Part model, mm, in its own coordinate system. A direction names the side the tool comes from. Coordinates: 2 decimals unless noted, no trailing zeros. Loops run counter-clockwise (first coordinate to the right, second up) from the corner with the lowest first, then second, coordinate; pieces in that order, holes last. Notation, with made-up numbers: M 79,29.5 L 111,29.5 A9 ccw 111,33.5 Z; hole C 35,39.5 d5. An arc over 180 degrees is marked long. Use a Markdown table: item, result. Add a question column.
1) Band-saw the part on D-D (y = 7.25). List the corners of the cut face in (x, z).
2) Band-saw the part on A-A (x = 0). List the corners of the cut face in (y, z), plus the area to 3 significant figures.
3) Pin check, flat tips, straight feed: pin 1 Ø1.5 at (y, z) = (7.5, -7) entering from +X; pin 2 Ø3 at (y, z) = (2.5, -3.5) entering from -X; pin 3 Ø4 at (x, z) = (0, -6.5) entering from +Y; pin 4 Ø4 at (x, z) = (0, 8.3) entering from +Y. Stop position of each tip, or through.
4) Pull direction Z, two halves, no side cores. Call faces 1 (the cylindrical face through (4.336, 8.874, 19.524)), 2 (the cylindrical face through (6.586, 15.042, -10.329)), 3 (the flat face through (13.42, 20, -5.25)): released by +Z, released by -Z, zero draft, split by the parting line, or undercut.
5) Band-saw the part on B-B (y = 14.75). List the corners of the cut face in (x, z), plus the area to 3 significant figures.
6) Wall check: probe 1 along Z at (x, y) = (0, 9); probe 2 along Z at (x, y) = (0, 15); probe 3 along X at (y, z) = (17.75, -0.5). Give the ranges that are in metal, low to high. Write a range as from..to.
7) Tool access for faces 4 (the cylindrical face through (-0.867, 15.944, -3.905)), 5 (the flat face through (0, 0, 0)): list every direction of +Z, -Z, +X, -X, +Y, -Y with a clear straight run to the whole face (end or side of a thin tool).
8) Band-saw the part on C-C (z = 0). List the corners of the cut face in (x, y), plus the area to 3 significant figures.
Autodesk Inventor part; units mm, degrees
ref_plane "YZ Plane" through (0, 0, 0) normal (1, 0, 0) x (0, 1, 0)
ref_plane "XZ Plane" through (0, 0, 0) normal (0, 1, 0) x (-1, 0, 0)
ref_plane "XY Plane" through (0, 0, 0) normal (0, 0, 1) x (1, 0, 0)
sketch "Sketch1" plane through (0, 0, 0) normal (0, 1, 0) x (-1, 0, 0)
  circle A0 centre (0, 0) radius 20
  dimension "d0" = 40
extrude "Extrusion1" add sketch "Sketch1" along normal blind 20
sketch "Sketch2" plane through (0, 20, 0) normal (0, 1, 0) x (1, 0, 0)
  circle A0 centre (0, 0) radius 12.25
  dimension "d3" = 24.5
extrude "Extrusion2" cut sketch "Sketch2" against normal blind 8
fillet "Fillet1" radius 2 2 edges at (20, 20, 0) (-12.25, 20, 0)
sketch "Sketch3" plane through (0, 12, 0) normal (0, 1, 0) x (1, 0, 0)
  circle A0 centre (0, 0) radius 4
  dimension "d7" = 8
extrude "Extrusion3" add sketch "Sketch3" along normal blind 8
sketch "Sketch4" plane through (0, 12, 0) normal (0, 1, 0) x (1, 0, 0)
  circle A0 centre (0, -8.3036) radius 2.5
  point P0 (0, 0)
  dimension "d10" = 5
extrude "Extrusion4" cut sketch "Sketch4" against normal blind 15
pattern_circular "Circular Pattern1" count 2 over 360 about axis through (0, -10, 0) along (0, 1, 0) of "Extrusion4"
properties part number "PruebaRodamiento"
Entries:
| question | item | result |
|---|---|---|
| 1 | outline | C 0,0 d40; hole C 0,-8.3 d5; hole C 0,8.3 d5 |
| 2 | outline | M 0,-20 L 18,-20 A2 ccw 20,-18 L 20,-14.25 A2 ccw 18,-12.25 L 12,-12.25 L 12,-10.8 L 0,-10.8 Z; M 0,-5.8 L 12,-5.8 L 12,-4 L 20,-4 L 20,4 L 12,4 L 12,5.8 L 0,5.8 Z; M 0,10.8 L 12,10.8 L 12,12.25 L 18,12.25 A2 ccw 20,14.25 L 20,18 A2 ccw 18,20 L 0,20 Z |
| 2 | area | 545 mm2 |
| 3 | pin 1 | x = 19 |
| 3 | pin 2 | x = -19.9 |
| 3 | pin 3 | y = 12 |
| 3 | pin 4 | through |
| 4 | face 1 | split by the parting line |
| 4 | face 2 | undercut |
| 4 | face 3 | zero draft |
| 5 | outline | C 0,0 d40; C 0,0 d8; hole C 0,0 d24.5 |
| 5 | area | 835 mm2 |
| 6 | probe 1 | -20..-10.8, -5.8..5.8, 10.8..20 |
| 6 | probe 2 | -20..-12.25, -4..4, 12.25..20 |
| 6 | probe 3 | -19.99..-12.24, -3.97..3.97, 12.24..19.99 |
| 7 | face 4 | +Y |
| 7 | face 5 | +Z, -Z, +X, -X, -Y |
| 8 | outline | M -20,0 L 20,0 L 20,18 A2 ccw 18,20 L 14.25,20 A2 ccw 12.25,18 L 12.25,12 L 4,12 L 4,20 L -4,20 L -4,12 L -12.25,12 L -12.25,18 A2 ccw -14.25,20 L -18,20 A2 ccw -20,18 Z |
| 8 | area | 665 mm2 |
